Input: part model. Units: mm. Frame: model coordinates. Face numbers are marked on the shaded views. A direction names the side the tool comes from. Coordinates: 2 decimals unless noted, no trailing zeros. Loops run counter-clockwise (first coordinate to the right, second up) from the corner with the lowest first, then second, coordinate; pieces in that order, holes last.
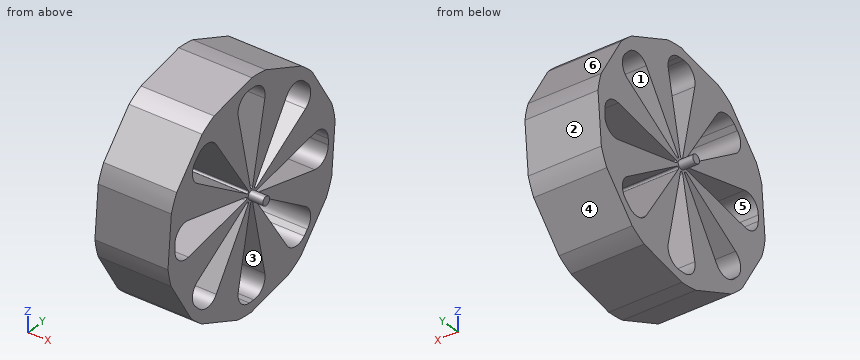
```python
from build123d import *

# Parameters (mm, degrees)
F0_R     = 37.5
F1_DEPTH = 12.5
F3_DEPTH = 12.5
F4_COUNT = 8
F6_DEPTH = 12.5
F7_R     = 1.5
F8_DEPTH = 17.5


with BuildPart() as f1:
    # F0 (on Right) → F1 (new body, symmetric)
    with BuildSketch(Plane.YZ):
        Circle(F0_R)
    extrude(amount=F1_DEPTH, both=True)

    # F2 (on Right) → F3 (cut, symmetric)
    with BuildSketch(Plane.YZ):
        with BuildLine():
            ThreePointArc((5.8991823905, 28.0400841101), (4.892101729, 32.223904361), (1.0076208802, 34.075760696))
            Line((1.0076208802, 34.075760696), (-1.0076208802, 34.075760696))
            ThreePointArc((-1.0076208802, 34.075760696), (-4.892101729, 32.223904361), (-5.8991823905, 28.0400841101))
            Line((-5.8991823905, 28.0400841101), (-0.489156151, 2.4882115641))
            ThreePointArc((-0.489156151, 2.4882115641), (0, 2.0917792227), (0.489156151, 2.4882115641))
            Line((0.489156151, 2.4882115641), (5.8991823905, 28.0400841101))
        make_face()
    f3 = extrude(amount=F3_DEPTH, both=True, mode=Mode.SUBTRACT)

    # F4: F3 ×8 about axis
    f4_axis = Axis((12.5, 0, 0), (1, 0, 0))
    for i in range(1, F4_COUNT):
        add(f3.rotate(f4_axis, i * 360 / F4_COUNT), mode=Mode.SUBTRACT)

    # F5 (on Right) → F6 (intersect, symmetric)
    with BuildSketch(Plane.YZ):
        Polygon((37.3855511828, 8.6729428424), (25.1477183542, 28.9912337848), (3.3043118538, 38.2358587972), (-19.8012294653, 32.8756853382), (-35.3433741477, 14.9581174833), (-37.3855511828, -8.6729428424), (-25.1477183542, -28.9912337848), (-3.3043118538, -38.2358587972), (19.8012294653, -32.8756853382), (35.3433741477, -14.9581174833), align=None)
    extrude(amount=F6_DEPTH, both=True, mode=Mode.INTERSECT)

    # F7 (on Right) → F8 (join, symmetric)
    with BuildSketch(Plane.YZ):
        Circle(F7_R)
    extrude(amount=F8_DEPTH, both=True)


solid = f1.part
```
Item 1: Mould query, pull axis Z, two halves, no side actions, for the marked faces 3, 4, 5 and 6. Classes: +Z half, -Z half, draft (parallel to the pull), parting line (faces both ways), or undercut.
Result:
face 3: undercut
face 4: -Z half
face 5: undercut
face 6: +Z half
Item 2: Line query: L1, parallel to Z at x = -9.5, y = -18.5; L2, parallel to Z at x = 2, y = 23; L3, parallel to Y at x = -9, z = 19. Output: solid intervals per line, ascending.
Result:
L1: z = -31.8 to -26.09, -12.08 to -3.88, 3.88 to 12.08, 26.09 to 32.62
L2: z = -29.19 to -25.15, -15.01 to -4.83, 4.83 to 15.01, 25.15 to 29.62
L3: y = -31.84 to -26.2, -12.4 to -3.99, 3.99 to 12.4, 26.2 to 31.17
Item 3: Section query A-A (x = 2). Count the separate pieces of the cut face and the enclosed holes in it, then the cut area to 3 significant figures.
Result:
separate pieces: 1
enclosed holes: 8
area: 2,500 mm2
Item 4: Contact query for flat-ended pins moving along their axis: P1, Ø5, axis at x = -6, y = 7.5, coming from the -Z side; P2, Ø12, axis at y = 21, z = 22, coming from the +X side; P3, Ø6, axis at x = 12.5, z = 18, coming from the -Y side; P4, Ø2, axis at y = 22.5, z = -16, coming from the +X side. Output: stop coordinate, or through.
Result:
P1: stops at z = -36.31
P2: stops at x = 12.5
P3: stops at y = -34.37
P4: passes through
Item 5: Reachability of the marked faces 1 and 2 from +Z, -Z, +X, -X, +Y, -Y: full face, straight path, thin tool, end or side. Return the list, or none.
Result:
face 1: +X, -X
face 2: -Z, +X, -X, +Y
Item 6: Section query B-B (z = 21). Output: boundary loops of the cut face in (x, y), then the cut area to 3 significant figures.
Result:
outline: (-12.5, -30.1) - (12.5, -30.1) - (12.5, -26.14) - (-12.5, -26.14) - close; (-12.5, -13.71) - (12.5, -13.71) - (12.5, -4.41) - (-12.5, -4.41) - close; (-12.5, 4.41) - (12.5, 4.41) - (12.5, 13.71) - (-12.5, 13.71) - close; (-12.5, 26.14) - (12.5, 26.14) - (12.5, 29.96) - (-12.5, 29.96) - close
area: 660 mm2
